Verification items for the finished model (mm, model axes). Round coordinates to 2 decimals unless told otherwise and drop trailing zeros. Write each loop counter-clockwise with the first axis right and the second up, starting at its lowest first coordinate (ties: lowest second). Pieces come first, ordered by that corner, then holes. Notation, with made-up numbers: M 17.5,80 L 64.5,80 A9 cw 64.5,90 Z; hole C 3,68 d4. An arc over 180 degrees is marked long. Write each question's results on one line, items separated by ' | '.
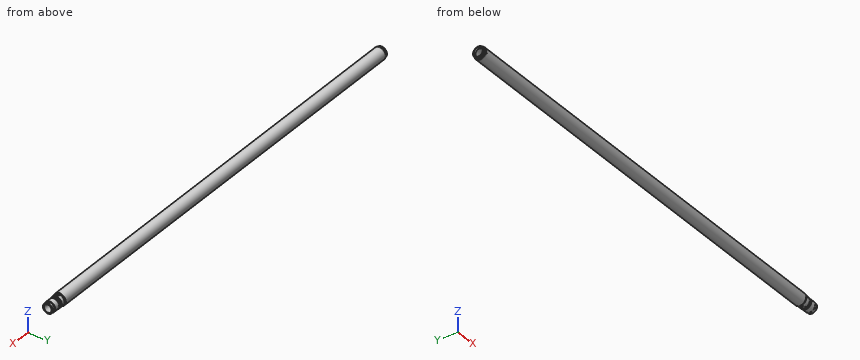
from build123d import *

# Parameters (mm, degrees)
SKETCH2_R                  = 4.5
F_9_GENNEMG_ENDE_HUL_DEPTH = 50


with BuildPart() as part:
    # Sketch1 → Base-Revolve (revolve)
    with BuildSketch(Plane.XY):
        with BuildLine():
            Line((0, 21), (0, 23.5))
            Line((0, 23.5), (0.5, 24))
            Line((0.5, 24), (5, 24))
            Line((5, 24), (5, 24.75))
            Line((5, 24.75), (7.5, 24.75))
            Line((7.5, 24.75), (11.830127019, 27.25))
            Line((11.830127019, 27.25), (17, 27.25))
            Line((17, 27.25), (17, 27.5))
            Line((17, 27.5), (1971.669872981, 27.5))
            Line((1971.669872981, 27.5), (1976, 25))
            Line((1976, 25), (1992.5, 25))
            ThreePointArc((1992.5, 25), (1992.853553391, 24.853553391), (1993, 24.5))
            Line((1993, 24.5), (1993, 23.5))
            Line((1993, 23.5), (1999, 23.5))
            Line((1999, 23.5), (1999, 24.5))
            ThreePointArc((1999, 24.5), (1999.146446609, 24.853553391), (1999.5, 25))
            Line((1999.5, 25), (2001, 25))
            Line((2001, 25), (2002, 24.422649731))
            Line((2002, 24.422649731), (2002, 23.75))
            ThreePointArc((2002, 23.75), (2002.292893219, 23.042893219), (2003, 22.75))
            Line((2003, 22.75), (2005, 22.75))
            Line((2005, 22.75), (2007.453263132, 24))
            Line((2007.453263132, 24), (2031.401923789, 24))
            Line((2031.401923789, 24), (2034, 22.5))
            Line((2034, 22.5), (2044, 22.5))
            Line((2044, 22.5), (2045, 21.922649731))
            Line((2045, 21.922649731), (2045, 17.5))
            Line((2045, 17.5), (6.062177826, 17.5))
            Line((6.062177826, 17.5), (0, 21))
        make_face()
    revolve(axis=Axis((0, 0, 0), (1, 0, 0)))

    # Sketch2 → ø9 gennemgående hul (cut, symmetric)
    with BuildSketch(Plane.XY):
        with Locations((1981, 0)):
            Circle(SKETCH2_R)
    extrude(amount=F_9_GENNEMG_ENDE_HUL_DEPTH, both=True, mode=Mode.SUBTRACT)


solid = part.part
1) Material ranges on line 1 (Z direction, x = 1035, y = -1); line 2 (Y direction, x = 250.5, z = 2); line 3 (Y direction, x = 1278, z = -5.5), recorded low to high. Write a range as [from, to].
Calculated:
line 1: z = [-27.48, -17.47], [17.47, 27.48] | line 2: y = [-27.43, -17.39], [17.39, 27.43] | line 3: y = [-26.94, -16.61], [16.61, 26.94]
2) Depth check by flat-ended pin: P1, Ø2, axis at x = 1567, y = -18, coming from the -Z side; P2, Ø11.5, axis at x = 1981, y = 0, coming from the +Z side; P3, Ø1, axis at x = 442, y = 0.5, coming from the -Z side; P4, Ø24.5, axis at y = 2.5, z = -2.5, coming from the +X side. Enter the tip coordinate at first touch or a pass-through.
Calculated:
P1: stops at z = -21.62 | P2: stops at z = 25.43 | P3: stops at z = -27.5 | P4: passes through
3) Sectioned sample at A-A, the plane x = 1332.5. Record the cut outline in (y, z), and give its area (3 significant figures).
Calculated:
outline: C 0,0 d55; hole C 0,0 d35 | area: 1,410 mm²
